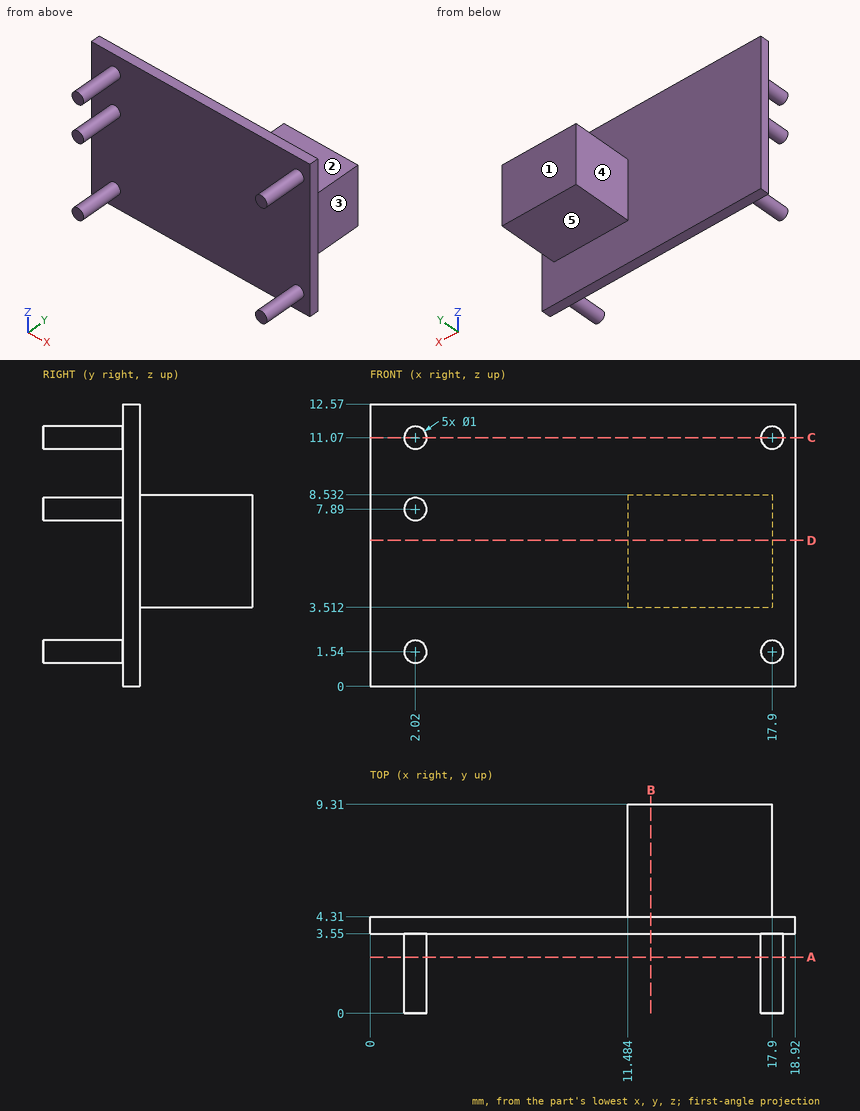
Geometry check sheet. Reference: drawing and pictorial views, mm from the part's lowest x, y, z. A direction names the side the tool comes from. Coordinates: 2 decimals unless noted, no trailing zeros. Order: outer loops, then holes, each group sorted by start corner. A loop starts at its lowest first (then second) coordinate and runs counter-clockwise, first axis right, second up. Notation, with made-up numbers: (-32.5, 20) - (-1.5, 20) arc R27 cw to (-1.5, 48) - close; hole circle Ø3 at (82.5, 70.5). An arc over 180 degrees is marked (long way). Answer in a Markdown table with one row per item. Add a question column.
1) Set-up check for the marked faces 1, 2, 3, 4 and 5: record each of +Z, -Z, +X, -X, +Y, -Y from which the full face is reachable in a straight line by a thin tool's end or side.
2) Cross-section at A-A, the plane y = 2.5. Record the cut outline in (x, z).
3) Cross-section at B-B, the plane x = 12.5. Record the cut outline in (y, z).
4) Material ranges on line 1 along X through (y, z) = (0.5, 11) (1 decimal); line 2 along X through (y, z) = (5.75, 7); line 3 along Y through (x, z) = (4.5, 1.5), recorded low to high. Write a range as [from, to].
5) Cross-section at C-C, the plane z = 11.07. Record the cut outline in (x, y).
6) Gauge pin test, flat ends, axial feed: P1, Ø2, axis at x = 5.5, z = 8.5, coming from the +Y side; P2, Ø1, axis at x = 16, y = 3, coming from the +Z side; P3, Ø4, axis at y = 7.5, z = 6.5, coming from the -X side; P4, Ø2.5, axis at x = 16, y = 6.5, coming from the -Z side. Record the tip position at first contact, or that the pin passes through.
7) Cross-section at D-D, the plane z = 6.5. Record the cut outline in (x, y).
Check result:
| question | item | result |
|---|---|---|
| 1 | face 1 | +Z, -Z, +X, -X, +Y |
| 1 | face 2 | +Z, +X, -X, +Y |
| 1 | face 3 | +Z, -Z, +X, +Y |
| 1 | face 4 | +Z, -Z, -X, +Y |
| 1 | face 5 | -Z, +X, -X, +Y |
| 2 | outline | circle Ø1 at (2.02, 1.54); circle Ø1 at (2.02, 7.89); circle Ø1 at (2.02, 11.07); circle Ø1 at (17.9, 1.54); circle Ø1 at (17.9, 11.07) |
| 3 | outline | (3.55, 0) - (4.31, 0) - (4.31, 3.51) - (9.31, 3.51) - (9.31, 8.53) - (4.31, 8.53) - (4.31, 12.57) - (3.55, 12.57) - close |
| 4 | line 1 | x = [1.5, 2.5], [17.4, 18.4] |
| 4 | line 2 | x = [11.48, 17.9] |
| 4 | line 3 | y = [3.55, 4.31] |
| 5 | outline | (0, 3.55) - (1.52, 3.55) - (1.52, 0) - (2.52, 0) - (2.52, 3.55) - (17.4, 3.55) - (17.4, 0) - (18.4, 0) - (18.4, 3.55) - (18.92, 3.55) - (18.92, 4.31) - (0, 4.31) - close |
| 6 | P1 | stops at y = 4.31 |
| 6 | P2 | passes through |
| 6 | P3 | stops at x = 11.48 |
| 6 | P4 | stops at z = 3.51 |
| 7 | outline | (0, 3.55) - (18.92, 3.55) - (18.92, 4.31) - (17.9, 4.31) - (17.9, 9.31) - (11.48, 9.31) - (11.48, 4.31) - (0, 4.31) - close |
